Check sheet for the modelled part. Datum: model origin and axes. Units: mm. A direction names the side the tool comes from. Round coordinates to 2 decimals unless told otherwise and drop trailing zeros. Write each loop counter-clockwise with the first axis right and the second up, starting at its lowest first coordinate (ties: lowest second). Pieces come first, ordered by that corner, then holes. Notation, with made-up numbers: (52.5, 5) -> (88.5, 5) arc R21 cw to (88.5, 25) -> close; hole circle Ø11 at (9, 60). An arc over 180 degrees is marked (long way). One line per item, written item: value. Start each with the question number.
```python
from build123d import *

# Parameters (mm, degrees)
F0_R     = 20
F1_DEPTH = 9
F2_R     = 3
F3_DEPTH = 9.001
F5_DEPTH = 4.25
F6_R     = 1.25
F7_DEPTH = 28.001


with BuildPart() as f1:
    # F0 (on Front) → F1 (new body)
    with BuildSketch(Plane.XZ):
        Circle(F0_R)
    extrude(amount=F1_DEPTH)

    # F2 (on face) → F3 (cut, through all)
    with BuildSketch(Plane.XZ.offset(9)):
        Circle(F2_R)
    extrude(amount=-F3_DEPTH, mode=Mode.SUBTRACT)

    # F4 (on Top) → F5 (join, symmetric)
    with BuildSketch(Plane.XY):
        with BuildLine():
            Line((15.483786, -9), (20, -9))
            Line((20, -9), (21, -9))
            ThreePointArc((21, -9), (23.12132, -9.87868), (24, -12))
            Line((24, -12), (24, -33.5))
            Line((24, -33.5), (28, -33.5))
            Line((28, -33.5), (28, -9))
            Line((28, -9), (28, 0))
            Line((28, 0), (20, 0))
            Line((20, 0), (15.483786, 0))
            Line((15.483786, 0), (15.483786, -9))
        make_face()
    extrude(amount=F5_DEPTH, both=True)

    # F6 (on Right) → F7 (cut, through all)
    with BuildSketch(Plane.YZ):
        with Locations((-26.25, 0)):
            Circle(F6_R)
    extrude(amount=F7_DEPTH, mode=Mode.SUBTRACT)


solid = f1.part
```
1. Release check for a two-part mould opening along Y. For faces 5 (the face through (4, 0, 0)), 6 (the face through (26, -25, 0)), 7 (the face through (-19.983, -4.437, 0.819)) record: +Y half, -Y half, draft (parallel to the pull), parting line (faces both ways), or undercut.
2. Cross-section at C-C (z = 0). Record the cut outline in (x, y).
3. Cross-section at B-B (y = -26.25). Record the cut outline in (x, z).
4. Access from +Z, -Z, +X, -X, +Y, -Y to the whole of each face (thin tool, end or side, straight path). Record for faces 1 (the face through (26, -33.5, 0)), 2 (the face through (25, -13, 4.25)), 3 (the face through (25, -13, -4.25)), 4 (the face through (24, -23, 0)).
5. Cross-section at D-D (y = -2.5). Record the cut outline in (x, z), plus the area to 3 significant figures.
6. Cross-section at A-A (x = 0). Record the cut outline in (y, z), plus the area to 3 significant figures.
7. Material ranges on probe 1 along Z at (x, y) = (0, -3); probe 2 along Y at (x, z) = (26, 0); probe 3 along Z at (x, y) = (25.65, -26.25), recorded low to high.
8. Depth check by flat-ended pin: pin 1 Ø2.5 at (y, z) = (-26, 1) entering from -X; pin 2 Ø4 at (x, y) = (14.5, -10.5) entering from +Z; pin 3 Ø3.5 at (x, z) = (0, 0) entering from +Y; pin 4 Ø5 at (x, z) = (3, 3.5) entering from -Y. Enter the tip coordinate at first touch or a pass-through.
Working result:
1. face 5: +Y half
1. face 6: undercut
1. face 7: draft
2. outline: (-20, -9) -> (-3, -9) -> (-3, 0) -> (-20, 0) -> close; (3, -9) -> (21, -9) arc R3 cw to (24, -12) -> (24, -25) -> (28, -25) -> (28, 0) -> (3, 0) -> close; (24, -33.5) -> (28, -33.5) -> (28, -27.5) -> (24, -27.5) -> close
3. outline: (24, -4.25) -> (28, -4.25) -> (28, -1.25) -> (24, -1.25) -> close; (24, 1.25) -> (28, 1.25) -> (28, 4.25) -> (24, 4.25) -> close
4. face 1: +Z, -Z, +X, -X, -Y
4. face 2: +Z, +X, +Y, -Y
4. face 3: -Z, +X, +Y, -Y
4. face 4: +Z, -Z, -X, -Y
5. outline: (19.54, -4.25) -> (28, -4.25) -> (28, 4.25) -> (19.54, 4.25) arc R20 ccw (long way) to start; hole circle Ø6 at (0, 0)
5. area: 1,300 mm^2
6. outline: (-9, -20) -> (0, -20) -> (0, -3) -> (-9, -3) -> close; (-9, 3) -> (0, 3) -> (0, 20) -> (-9, 20) -> close
6. area: 306 mm^2
7. probe 1: z = -20 to -3, 3 to 20
7. probe 2: y = -33.5 to -27.5, -25 to 0
7. probe 3: z = -4.25 to -1.25, 1.25 to 4.25
8. pin 1: stops at x = 24
8. pin 2: stops at z = 15.05
8. pin 3: passes through
8. pin 4: stops at y = -9
